Design review of the part built by this model. Coordinates are the model's own, in mm. A direction names the side the tool comes from. Round coordinates to 2 decimals unless told otherwise and drop trailing zeros. Loops run counter-clockwise (first coordinate to the right, second up) from the corner with the lowest first, then second, coordinate; pieces in that order, holes last. Notation, with made-up numbers: (-18, 48) - (-3, 48) arc R17 ccw to (-3, 63) - close; hole circle Ø3 at (58, 83.5). An arc over 180 degrees is marked (long way). Answer as CSV lines item,"result". Start each with the question number.
(1) Wall thickness on L1, parallel to Y at x = -100.5, z = -3.75; L2, parallel to Z at x = 48, y = 22; L3, parallel to Z at x = 106.5, y = -8: over which ranges is each line inside the solid? List them lowest first.
(2) For P1, Ø1, axis at x = -98, z = -8, coming from the +Y side; P2, Ø1.5, axis at x = -48.5, z = -6.5, coming from the +Y side; P3, Ø0.7, axis at x = -11.5, z = -3, coming from the +Y side; P4, Ø1, axis at y = 17, z = -5.5, coming from the +X side, all flat-tipped, find the tip position at first contact; note any pin that passes through.
(3) Consider section D-D (y = -42.5). Give the boundary of the cut face in (x, z) (3 decimals).
(4) Consider section A-A (x = -117.5). Give the boundary of the cut face in (y, z).
(5) Consider section B-B (y = 13). Give the boundary of the cut face in (x, z) (3 decimals), and give its area (3 significant figures).
(6) Consider section C-C (y = -11). Give the boundary of the cut face in (x, z) (3 decimals), and give its area (3 significant figures).
(7) For faces 4 (the flat face through (1, 16, -7.396)), 5 (the flat face through (41, 18, -8.646)), 6 (the flat face through (-149.225, -22, -7)), list the 3-axis set-ups (+Z, -Z, +X, -X, +Y, -Y) from which the entire face can be reached by the end or side of a thin tool; tool diameter is ignored.
(8) Mouldability with a two-part tool opening along X and no side actions: class faces 1 (the flat face through (1, -39, -4.396)), 2 (the cylindrical face through (-146.819, 27.097, -9.326)), 3 (the flat face through (-92, 18, -8.646)) as released by +X, released by -X, zero draft, split by the parting line, or undercut.
from build123d import *

# Parameters (mm, degrees)
BOSS_EXTRUDE1_DEPTH = 304.800275
FILLET1_R           = 8
SKETCH2_W           = 38.10085
SKETCH2_H           = 23.904524524
SKETCH2_W_2         = 38.1
CUT_EXTRUDE1_DEPTH  = 1.25
FILLET2_R           = 1.6
FILLET3_R           = 1.6


with BuildPart() as part:
    # Sketch1 → Boss-Extrude1 (new body)
    with BuildSketch(Plane.ZY.offset(149.225)):
        Polygon((-2, -64.3742065), (-3.3962, -64.3742065), (-3.3962, -50.048837521), (-4.3962, -50.048837521), (-4.3962, -28.126347), (-5.3962, -28.126347), (-5.3962, 3.873653), (-7.3962, 3.873653), (-7.3962, 29.378177524), (-11.202667042, 29.378177524), (-4, -73.62476), (-2, -73.62476), align=None)
    extrude(amount=-BOSS_EXTRUDE1_DEPTH)

    # Fillet1
    fillet1_edges = [part.edges().sort_by_distance(p)[0] for p in [
        (-149.225, 29.378177524, -9.299433521),
        (155.575275, 29.378177524, -9.299433521),
    ]]
    fillet(fillet1_edges, radius=FILLET1_R)

    # Sketch2 → Cut-Extrude1 (cut)
    with BuildSketch(Plane.XY.offset(-7.3962)):
        with Locations((41.2757, 17.425915262)):
            Rectangle(SKETCH2_W, SKETCH2_H)
        with Locations((-92.074875, 17.425915262)):
            Rectangle(SKETCH2_W_2, SKETCH2_H)
        with Locations((-34.92515, 17.425915262)):
            Rectangle(SKETCH2_W, SKETCH2_H)
        with Locations((98.425425, 17.425915262)):
            Rectangle(SKETCH2_W_2, SKETCH2_H)
    extrude(amount=-CUT_EXTRUDE1_DEPTH, mode=Mode.SUBTRACT)

    # Fillet2
    fillet2_edges = [part.edges().sort_by_distance(p)[0] for p in [
        (-111.124875, 5.473653, -8.0212),
        (-73.024875, 5.473653, -8.0212),
        (-53.975575, 5.473653, -8.0212),
        (-15.874725, 5.473653, -8.0212),
        (60.326125, 5.473653, -8.0212),
        (22.225275, 5.473653, -8.0212),
        (117.475425, 5.473653, -8.0212),
        (79.375425, 5.473653, -8.0212),
    ]]
    fillet(fillet2_edges, radius=FILLET2_R)

    # Fillet3
    fillet3_edges = [part.edges().sort_by_distance(p)[0] for p in [
        (-111.124875, 29.378177524, -8.0212),
        (-73.024875, 29.378177524, -8.0212),
        (-53.975575, 29.378177524, -8.0212),
        (-15.874725, 29.378177524, -8.0212),
        (22.225275, 29.378177524, -8.0212),
        (60.326125, 29.378177524, -8.0212),
        (79.375425, 29.378177524, -8.0212),
        (117.475425, 29.378177524, -8.0212),
    ]]
    fillet(fillet3_edges, radius=FILLET3_R)


solid = part.part
Determined:
1,L1,"y = -73.62 to -50.05"
1,L2,"z = -10.69 to -8.65"
1,L3,"z = -8.59 to -5.4"
2,P1,"stops at y = 5.47"
2,P2,"stops at y = 3.87"
2,P3,"stops at y = -64.37"
2,P4,"passes through"
3,outline,"(-149.225, -6.176) - (155.575, -6.176) - (155.575, -4.396) - (-149.225, -4.396) - close"
4,outline,"(-73.62, -4) - (29.38, -11.2) - (29.38, -7.4) - (3.87, -7.4) - (3.87, -5.4) - (-28.13, -5.4) - (-28.13, -4.4) - (-50.05, -4.4) - (-50.05, -3.4) - (-64.37, -3.4) - (-64.37, -2) - (-73.62, -2) - close"
5,outline,"(-149.225, -10.057) - (155.575, -10.057) - (155.575, -7.396) - (117.475, -7.396) - (117.475, -8.646) - (79.375, -8.646) - (79.375, -7.396) - (60.326, -7.396) - (60.326, -8.646) - (22.225, -8.646) - (22.225, -7.396) - (-15.875, -7.396) - (-15.875, -8.646) - (-53.976, -8.646) - (-53.976, -7.396) - (-73.025, -7.396) - (-73.025, -8.646) - (-111.125, -8.646) - (-111.125, -7.396) - (-149.225, -7.396) - close"
5,area,"621 mm^2"
6,outline,"(-149.225, -8.379) - (155.575, -8.379) - (155.575, -5.396) - (-149.225, -5.396) - close"
6,area,"909 mm^2"
7,face 4,"+Z, +X, -X, +Y"
7,face 5,"+Z, +Y"
7,face 6,"+Z, -Z, -X, +Y, -Y"
8,face 1,"zero draft"
8,face 2,"released by -X"
8,face 3,"undercut"
